Input: part model. Units: mm. Frame: model coordinates. Face numbers are marked on the shaded views. A direction names the side the tool comes from. Coordinates: 2 decimals unless noted, no trailing zeros. Order: outer loops, then holes, each group sorted by start corner. A loop starts at its lowest first (then second) coordinate and runs counter-clockwise, first axis right, second up. Notation, with made-up numbers: (-8.5, 67.5) -> (8.5, 67.5) arc R31 cw to (8.5, 94.5) -> close; hole circle Ø1 at (4, 34.25). An arc over 180 degrees is marked (long way). Answer as CSV lines item,"result".
from build123d import *

# Parameters (mm, degrees)
F2_DEPTH = 14.986
F3_DEPTH = 14.478


with BuildPart() as f2:
    # F1 (on Right) → F2 (new body)
    with BuildSketch(Plane.YZ):
        Polygon((-143.724723, 81.765599), (1.051276, -165.352061), (142.673448, 83.586462), align=None)
    extrude(amount=F2_DEPTH)

    # F0 (on Front) → F3 (join)
    with BuildSketch(Plane.XZ):
        Polygon((44.456244, -53.21716), (64.350262, 25.835394), (-4.685595, 69.184312), (-67.246119, 16.922862), (-36.874792, -58.725407), align=None)
    extrude(amount=F3_DEPTH)


solid = f2.part
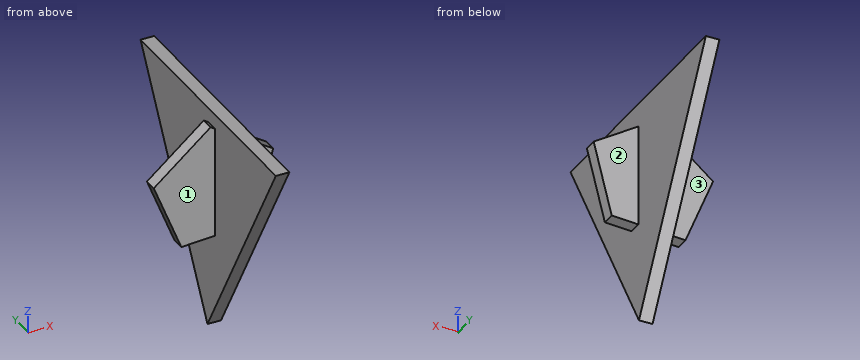
1. Cut plane A-A (z = 30.5). Return the cut outline in (x, y), plus the area to 3 significant figures.
Findings:
outline,"(-50.99, -14.48) -> (0, -14.48) -> (0, -113.69) -> (14.99, -113.69) -> (14.99, -14.48) -> (56.92, -14.48) -> (56.92, 0) -> (14.99, 0) -> (14.99, 112.47) -> (0, 112.47) -> (0, 0) -> (-50.99, 0) -> close"
area,"4,730 mm2"
2. Reachability of the marked faces 1, 2 and 3 from +Z, -Z, +X, -X, +Y, -Y: full face, straight path, thin tool, end or side. Return the list, or none.
Findings:
face 1,"+Z, -Z, -X, -Y"
face 2,"+Z, -Z, +X, +Y"
face 3,"+Z, -Z, -X, +Y"
3. Cut plane B-B (x = 10). Return the cut outline in (y, z), plus the area to 3 significant figures.
Findings:
outline,"(-143.72, 81.77) -> (1.05, -165.35) -> (142.67, 83.59) -> close"
area,"35,500 mm2"
4. Ray query, line 1 along Y through (x, z) = (41.5, -51.5); line 2 along X through (y, z) = (-2, 69); line 3 along X through (y, z) = (54.5, 14). Return the intervals inside material, ascending.
Findings:
line 1,"y = -14.48 to 0"
line 2,"x = -4.91 to -4.39, 0 to 14.99"
line 3,"x = 0 to 14.99"
5. Contact query for flat-ended pins moving along their axis: pin 1 (24.5 mm diameter, centred on x = 28, z = 17, fed in from +Y); pin 2 (3 mm diameter, centred on x = 13, z = -137.5, fed in from +Y); pin 3 (1.5 mm diameter, centred on y = 86, z = 12.5, fed in from +X). Output: stop coordinate, or through.
Findings:
pin 1,"stops at y = 0"
pin 2,"stops at y = 17.75"
pin 3,"stops at x = 14.99"
6. Cut plane D-D (z = -40). Return the cut outline in (x, y), plus the area to 3 significant figures.
Findings:
outline,"(-44.39, -14.48) -> (0, -14.48) -> (0, -72.39) -> (14.99, -72.39) -> (14.99, -14.48) -> (47.78, -14.48) -> (47.78, 0) -> (14.99, 0) -> (14.99, 72.36) -> (0, 72.36) -> (0, 0) -> (-44.39, 0) -> close"
area,"3,290 mm2"
7. Cut plane C-C (y = 25). Return the cut outline in (x, z).
Findings:
outline,"(0, -123.26) -> (14.99, -123.26) -> (14.99, 82.84) -> (0, 82.84) -> close"
